Could you check a few things on this model? Use its own coordinates, in mm. A direction names the side the tool comes from. Coordinates: 2 decimals unless noted, no trailing zeros.
```python
from build123d import *

# Parameters (mm, degrees)
SKETCH1_W           = 146.05
SKETCH1_H           = 19.05
BOSS_EXTRUDE1_DEPTH = 15.24
CUT_EXTRUDE5_DEPTH  = 1.905
CUT_EXTRUDE2_DEPTH  = 19.05
CUT_EXTRUDE3_DEPTH  = 149.073504166
SKETCH5_W           = 6.985
SKETCH5_H           = 3.81
CUT_EXTRUDE4_DEPTH  = 6.35


with BuildPart() as part:
    # Sketch1 → Boss-Extrude1 (new body)
    with BuildSketch(Plane(origin=(0, 0, 0), x_dir=(1, 0, 0), z_dir=(0, 1, 0))):
        with Locations((73.025, 9.525)):
            Rectangle(SKETCH1_W, SKETCH1_H)
    extrude(amount=BOSS_EXTRUDE1_DEPTH)

    # Sketch6 → Cut-Extrude5 (cut)
    with BuildSketch(Plane(origin=(0, 15.24, 0), x_dir=(1, 0, 0), z_dir=(0, 1, 0))):
        Polygon((5.792025279, 11.011495693), (7.429845792, 7.511495693), (6.969208773, 7.511495693), (6.437758452, 8.633290564), (5.006067747, 8.633290564), (4.474617426, 7.511495693), (4.019589382, 7.511495693), (5.65180092, 11.011495693), align=None)
        Polygon((5.7219131, 10.246571814), (5.177141465, 9.037136718), (6.272293709, 9.037136718), align=None, mode=Mode.SUBTRACT)
    extrude(amount=-CUT_EXTRUDE5_DEPTH, mode=Mode.SUBTRACT)

    # Sketch4 → Cut-Extrude2 (cut)
    with BuildSketch(Plane(origin=(0, 15.24, 0), x_dir=(1, 0, 0), z_dir=(0, 1, 0))):
        with BuildLine():
            add(Edge.make_bspline(
                [(4.476723392, 0), (17.725756487, 4.043101895), (17.090749047, 12.999753789), (25.262791442, 14.373397692), (26.219517358, 14.465775476)],
                knots=[0, 0, 0, 0, 0.256127126, 0.284585695, 0.284585695, 0.284585695, 0.284585695], degree=3))
            Line((4.476723392, 0), (142.875, 0))
            add(Edge.make_bspline(
                [(68.923918907, 14.861089556), (81.075041449, 14.855684794), (98.246564786, 14.797098309), (108.068516517, 14.713978549), (127.226778846, 16.049688466), (142.875, 0)],
                knots=[0.488488537, 0.488488537, 0.488488537, 0.488488537, 0.629203286, 0.700744717, 1, 1, 1, 1], degree=3))
            Line((68.923918907, 14.861089556), (26.219517358, 14.465775476))
        make_face()
        with BuildLine():
            add(Edge.make_bspline(
                [(105.157866441, 19.05), (131.491281961, 18.918345897), (139.296835945, 6.588803862), (146.05, 0)],
                knots=[0.010622627, 0.010622627, 0.010622627, 0.010622627, 1, 1, 1, 1], degree=3))
            Line((146.05, 0), (146.05, 19.05))
            Line((146.05, 19.05), (105.157866441, 19.05))
        make_face()
    extrude(amount=-CUT_EXTRUDE2_DEPTH, mode=Mode.SUBTRACT)

    # Sketch3 → Cut-Extrude3 (cut, through all)
    with BuildSketch(Plane(origin=(0, 0, -19.05), x_dir=(-1, 0, 0), z_dir=(0, 0, -1))):
        with BuildLine():
            Line((0, 0), (0, 8.89))
            add(Edge.make_bspline(
                [(0, 8.89), (-26.792555724, 10.094357911), (-71.276383534, 7.213998552), (-114.960678795, 0.591225669), (-132.239266272, 0)],
                knots=[0, 0, 0, 0, 0.551607579, 0.905919639, 0.905919639, 0.905919639, 0.905919639], degree=3))
            Line((-132.239266272, 0), (0, 0))
        make_face()
        with BuildLine():
            add(Edge.make_bspline(
                [(0, 15.24), (-48.91510465, 14.281311131), (-97.188371336, 5.218004406), (-146.05, 3.81)],
                knots=[0, 0, 0, 0, 1, 1, 1, 1], degree=3))
            Line((0, 15.24), (-146.05, 15.24))
            Line((-146.05, 15.24), (-146.05, 3.81))
        make_face()
    extrude(amount=-CUT_EXTRUDE3_DEPTH, mode=Mode.SUBTRACT)

    # Sketch5 → Cut-Extrude4 (cut)
    with BuildSketch(Plane.ZY):
        with Locations((-9.2075, 10.795)):
            Rectangle(SKETCH5_W, SKETCH5_H)
    extrude(amount=-CUT_EXTRUDE4_DEPTH, mode=Mode.SUBTRACT)


solid = part.part
```
1. If we mould it in two halves opening along Z, with no side actions, what happens to faces 3 (the face through (2, 12, 0)), 4 (the face through (3, 12.7, -9)), 5 (the face through (138, 0, -6)), 6 (the face through (5.73, 13.335, -8.88))? For each: pulls with the +Z half, pulls with the -Z half, needs draft (parallel to the pull), parting line crosses it, or undercut.
Verdict:
face 3: pulls with the +Z half
face 4: undercut
face 5: needs draft
face 6: undercut
2. On a 3-axis mill with a long thin cutter (end or side, diameter ignored), from which of +Z, -Z, +X, -X, +Y, -Y can I reach the whole of each face in a straight line? I mean faces 1 (the face through (0, 13, -9)), 2 (the face through (3, 11, -12.7)). Say none if no direction works.
Verdict:
face 1: +Z, -Z, -X, +Y, -Y
face 2: -X, -Y
3. Please list where these lines run through material, in increasing order: line 1 along Z through (x, y) = (27, 13); line 2 along X through (y, z) = (12.5, -7.75); line 3 along Y through (x, z) = (114.5, -16.25).
Verdict:
line 1: z = -19.05 to -14.47
line 2: x = 6.35 to 16.55
line 3: y = 1.21 to 5.63
4. For pin 1 (8 mm diameter, centred on x = 91.5, y = 13.5, fed in from +Z); pin 2 (3 mm diameter, centred on x = 2, z = -9, fed in from -Y); pin 3 (1.8 mm diameter, centred on y = 11.5, z = -8, fed in from -X); pin 4 (3 mm diameter, centred on x = 80, z = -14.5, fed in from -Y), each with a flat end and sliding along its axis, tell me the tip position at first contact or that it passes through.
Verdict:
pin 1: passes through
pin 2: stops at y = 12.7
pin 3: stops at x = 6.35
pin 4: stops at y = 5.11
